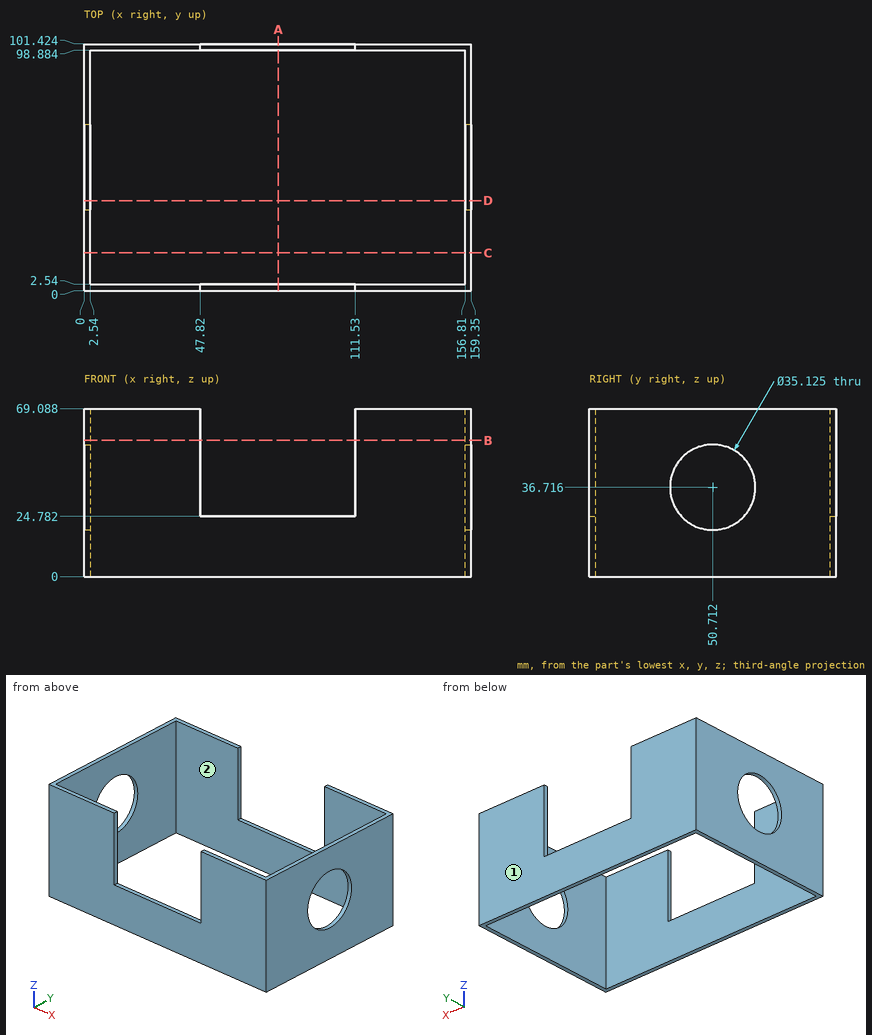
Study the drawing (mm; zero at the part's minimum x, y, z) and answer. A direction names the side the tool comes from. Coordinates: 2 decimals unless noted, no trailing zeros. Write each loop counter-clockwise with the first axis right and the second up, starting at its lowest first coordinate (ties: lowest second). Pieces come first, ordered by that corner, then holes. Notation, with made-up numbers: M -11,37 L -1,37 A19 ccw -1,45 Z; hole C -28,-29 d5. An arc over 180 degrees is marked long. Use a Markdown table: item, result. Add a question column.
1. Section B-B (z = 56) is taken. Give the vertices of the cut face in (x, y).
2. Section A-A (x = 80) is taken. Give the vertices of the cut face in (y, z).
3. Straight lines are drawn through the part: line 1 along Y through (x, z) = (47.5, 43); line 2 along X through (y, z) = (77, 21). For each, find the intervals that lie inside material, in ascending order. Write a range as [from, to].
4. Given P1, Ø6, axis at x = 88.5, z = 9, coming from the -Y side; P2, Ø3, axis at x = 78, y = 1, coming from the +Z side; P3, Ø21, axis at y = 50.71, z = 36.72, coming from the -X side, each flat-ended and moving along its own axis, determine where each tip first touches the part or whether it passes through.
5. Which of the six approach directions +Z, -Z, +X, -X, +Y, -Y give full straight-line access (tool end or side, diameter ignored) to the marked faces 1 and 2?
6. Section D-D (y = 37) is taken. Give the vertices of the cut face in (x, z).
7. Section C-C (y = 15.5) is taken. Give the vertices of the cut face in (x, z).
Data:
| question | item | result |
|---|---|---|
| 1 | outline | M 0,0 L 47.82,0 L 47.82,2.54 L 2.54,2.54 L 2.54,98.88 L 47.82,98.88 L 47.82,101.42 L 0,101.42 Z; M 111.53,0 L 159.35,0 L 159.35,101.42 L 111.53,101.42 L 111.53,98.88 L 156.81,98.88 L 156.81,2.54 L 111.53,2.54 Z |
| 2 | outline | M 0,0 L 2.54,0 L 2.54,24.78 L 0,24.78 Z; M 98.88,0 L 101.42,0 L 101.42,24.78 L 98.88,24.78 Z |
| 3 | line 1 | y = [0, 2.54], [98.88, 101.42] |
| 3 | line 2 | x = [0, 2.54], [156.81, 159.35] |
| 4 | P1 | stops at y = 0 |
| 4 | P2 | stops at z = 24.78 |
| 4 | P3 | passes through |
| 5 | face 1 | +Z, -Z, +X, -X, +Y |
| 5 | face 2 | +Z, -Z |
| 6 | outline | M 0,0 L 2.54,0 L 2.54,25.74 L 0,25.74 Z; M 0,47.69 L 2.54,47.69 L 2.54,69.09 L 0,69.09 Z; M 156.81,0 L 159.35,0 L 159.35,25.74 L 156.81,25.74 Z; M 156.81,47.69 L 159.35,47.69 L 159.35,69.09 L 156.81,69.09 Z |
| 7 | outline | M 0,0 L 2.54,0 L 2.54,69.09 L 0,69.09 Z; M 156.81,0 L 159.35,0 L 159.35,69.09 L 156.81,69.09 Z |
